Autodesk Inventor part; units mm, degrees
ref_plane "YZ Plane" through (0, 0, 0) normal (1, 0, 0) x (0, 1, 0)
ref_plane "XZ Plane" through (0, 0, 0) normal (0, 1, 0) x (-1, 0, 0)
ref_plane "XY Plane" through (0, 0, 0) normal (0, 0, 1) x (1, 0, 0)
sketch "Electronics box bottom layout" plane through (0, 0, 0) normal (0, 1, 0) x (-1, 0, 0)
  line L0 (-111.125, 304.8) -> (111.125, 304.8)
  line L1 (111.125, 304.8) -> (111.125, -304.8)
  line L2 (111.125, -304.8) -> (-111.125, -304.8)
  line L3 (-111.125, -304.8) -> (-111.125, 304.8)
  line L4 (-111.125, 304.8) -> (111.125, -304.8) construction
  line L5 (111.125, 304.8) -> (-111.125, -304.8) construction
  line L6 (-85.725, 304.8) -> (85.725, 304.8)
  line L7 (85.725, 304.8) -> (85.725, 330.2)
  line L8 (85.725, 330.2) -> (-85.725, 330.2)
  line L9 (-85.725, 330.2) -> (-85.725, 304.8)
  line L10 (-85.725, 304.8) -> (85.725, 330.2) construction
  line L11 (85.725, 304.8) -> (-85.725, 330.2) construction
  line L12 (85.725, -304.8) -> (-85.725, -304.8)
  line L13 (-85.725, -304.8) -> (-85.725, -330.2)
  line L14 (-85.725, -330.2) -> (85.725, -330.2)
  line L15 (85.725, -330.2) -> (85.725, -304.8)
  line L16 (85.725, -304.8) -> (-85.725, -330.2) construction
  line L17 (-85.725, -304.8) -> (85.725, -330.2) construction
  point P0 (0, 0)
  point P1 (0, 317.5)
  point P2 (0, -317.5)
  point P3 (-85.725, 304.8)
  dimension "d0" = 222.25
  dimension "d1" = 609.6
  dimension "d2" = 171.45
  dimension "d3" = 171.45
  dimension "d4" = 25.4
  dimension "d5" = 25.4
extrude "Base" add sketch "Electronics box bottom layout" along normal blind 1.5875
sketch "Sketch2" plane through (0, 1.5875, 0) normal (0, 1, 0) x (1, 0, 0)
  line L0 (-111.125, -304.8) -> (-85.725, -304.8)
  line L1 (-85.725, -304.8) -> (-85.725, -330.2)
  line L2 (-85.725, -330.2) -> (85.725, -330.2)
  line L3 (85.725, -330.2) -> (85.725, -304.8)
  line L4 (85.725, -304.8) -> (111.125, -304.8)
  line L5 (111.125, -304.8) -> (111.125, 304.8)
  line L6 (111.125, 304.8) -> (85.725, 304.8)
  line L7 (85.725, 304.8) -> (85.725, 330.2)
  line L8 (85.725, 330.2) -> (-85.725, 330.2)
  line L9 (-85.725, 330.2) -> (-85.725, 304.8)
  line L10 (-85.725, 304.8) -> (-111.125, 304.8)
  line L11 (-111.125, 304.8) -> (-111.125, -304.8)
  line L12 (-109.5375, -303.2125) -> (-84.1375, -303.2125)
  line L13 (-84.1375, -303.2125) -> (-84.1375, -328.6125)
  line L14 (-84.1375, -328.6125) -> (84.1375, -328.6125)
  line L15 (84.1375, -328.6125) -> (84.1375, -303.2125)
  line L16 (84.1375, -303.2125) -> (109.5375, -303.2125)
  line L17 (109.5375, -303.2125) -> (109.5375, 303.2125)
  line L18 (109.5375, 303.2125) -> (84.1375, 303.2125)
  line L19 (84.1375, 303.2125) -> (84.1375, 328.6125)
  line L20 (84.1375, 328.6125) -> (-84.1375, 328.6125)
  line L21 (-84.1375, 328.6125) -> (-84.1375, 303.2125)
  line L22 (-84.1375, 303.2125) -> (-109.5375, 303.2125)
  line L23 (-109.5375, 303.2125) -> (-109.5375, -303.2125)
  point P0 (0, 0)
  dimension "d8" = 1.5875
extrude "Walls" add sketch "Sketch2" along normal blind 61.9125
sketch "Sketch3" plane through (-85.725, 0, -330.2) normal (-1, 0, 0) x (0, 0, 1)
  line L0 (0, 63.5) -> (25.4, 63.5)
  line L1 (0, 0) -> (25.4, 0)
  line L2 (0, 0) -> (0, 63.5)
  point P0 (330.2, 0)
  point P1 (12.7, 38.1)
  point P2 (12.7, 12.7)
  dimension "d11" = 25.4
  dimension "d12" = 12.7
  dimension "d31" = 12.7
  dimension "d32" = 12.7
hole "Hole1" at (-85.725, 38.1, -317.5) at (-85.725, 12.7, -317.5) direction (1, 0, 0) diameter 6.35 end through all
sketch "Sketch4" plane through (-85.725, 0, -304.8) normal (0, 0, -1) x (-1, 0, 0)
  line L0 (0, 63.5) -> (25.4, 63.5)
  line L1 (25.4, 0) -> (25.4, 63.5)
  line L2 (0, 0) -> (25.4, 0)
  point P0 (-85.725, 0)
  point P1 (12.7, 38.1)
  point P2 (12.7, 12.7)
  dimension "d20" = 25.4
  dimension "d21" = 12.7
  dimension "d22" = 12.7
  dimension "d23" = 12.7
hole "Hole2" at (-98.425, 38.1, -304.8) at (-98.425, 12.7, -304.8) direction (0, 0, 1) diameter 6.35 end through all
pattern_linear "Rectangular Pattern1" count 2 spacing 635 along (0, 0, 1) of "Hole1"
pattern_linear "Rectangular Pattern2" count 2 spacing 196.85 along (1, 0, 0) of "Hole2"
equation "\"d2\" = d0 - 2 * d4"
equation "\"d3\" = d2"
equation "\"d5\" = d4"
properties part number "EBox-Frame" material "Air"
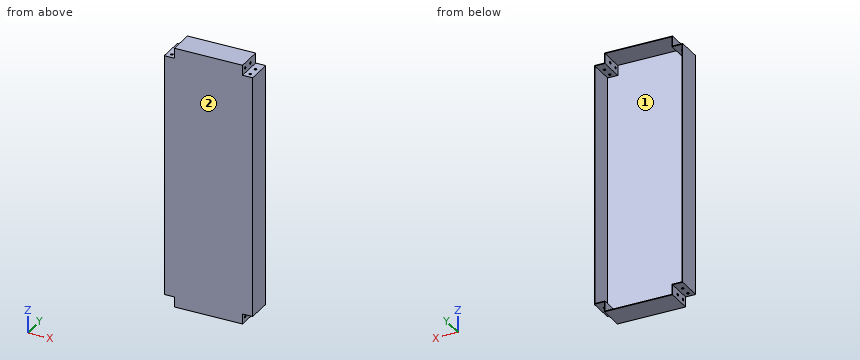
Design review of the part built by this model. Coordinates are the model's own, in mm. Face numbers are marked on the shaded views. Coordinates: 2 decimals unless noted, no trailing zeros. Order: outer loops, then holes, each group sorted by start corner. A loop starts at its lowest first (then second) coordinate and runs counter-clockwise, first axis right, second up. Notation, with made-up numbers: M -31,-22.5 L 14,-22.5 A33 ccw 14,10.5 Z; hole C 31.5,44.5 d2. An arc over 180 degrees is marked long. Answer as a JSON object with one key per item and string values. Group by question number.
1) Wall thickness on L1, parallel to Z at x = -85.2, y = 12.7 (1 decimal); L2, parallel to X at y = 46, z = -168 (1 decimal); L3, parallel to Z at x = 73, y = 57: over which ranges is each line inside the solid? List them lowest first.
2) Add section A-A, the plane x = -8.5. Write out the cut boundary in (y, z), then the cut area to 3 significant figures.
3) For pin 1 (8 mm diameter, centred on x = 29.5, z = -78.5, fed in from +Y); pin 2 (7.5 mm diameter, centred on x = -95.5, y = 41.5, fed in from +Z); pin 3 (12.5 mm diameter, centred on y = 19.5, z = 317, fed in from -X) (3 decimals), all flat-tipped, find the tip position at first contact; note any pin that passes through.
4) Add section C-C, the plane z = -124. Write out the cut boundary in (x, y) (1 decimal).
5) Mouldability with a two-part tool opening along X and no side actions: class the marked faces 1 and 2 as pulls with the +X half, pulls with the -X half, needs draft (parallel to the pull), parting line crosses it, or undercut.
6) Add section B-B, the plane y = 53.5. Write out the cut boundary in (x, z) (1 decimal), then the cut area to 3 significant figures.
Computed values:
{
 "1": {"L1": "z = -330.2 to -320.7, -314.3 to -303.2, 303.2 to 314.3, 320.7 to 330.2", "L2": "x = -111.1 to -109.5, 109.5 to 111.1", "L3": "z = -330.2 to -328.61, 328.61 to 330.2"},
 "2": {"outline": "M 0,-330.2 L 63.5,-330.2 L 63.5,-328.61 L 1.59,-328.61 L 1.59,328.61 L 63.5,328.61 L 63.5,330.2 L 0,330.2 Z", "area": "1,240 mm^2"},
 "3": {"pin 1": "stops at y = 1.59", "pin 2": "stops at z = 304.8", "pin 3": "stops at x = -85.725"},
 "4": {"outline": "M -111.1,0 L 111.1,0 L 111.1,63.5 L 109.5,63.5 L 109.5,1.6 L -109.5,1.6 L -109.5,63.5 L -111.1,63.5 Z"},
 "5": {"face 1": "undercut", "face 2": "needs draft"},
 "6": {"outline": "M -111.1,-304.8 L -85.7,-304.8 L -85.7,-330.2 L 85.7,-330.2 L 85.7,-304.8 L 111.1,-304.8 L 111.1,304.8 L 85.7,304.8 L 85.7,330.2 L -85.7,330.2 L -85.7,304.8 L -111.1,304.8 Z; hole M -109.5,-303.2 L -84.1,-303.2 L -84.1,-328.6 L 84.1,-328.6 L 84.1,-303.2 L 109.5,-303.2 L 109.5,303.2 L 84.1,303.2 L 84.1,328.6 L -84.1,328.6 L -84.1,303.2 L -109.5,303.2 Z", "area": "2,790 mm^2"}
}
